Here's how the part is built. I have some questions about the finished solid (model axes, mm). Face numbers are marked on the shaded views. A direction names the side the tool comes from. Give positions to 0.01 mm unless a question says otherwise; leave off trailing zeros. Loops run counter-clockwise (first coordinate to the right, second up) from the corner with the lowest first, then second, coordinate; pieces in that order, holes last. Notation, with made-up numbers: M -25,0 L 24,0 A15 ccw 24,5 Z; hole C -4,76 d8. An arc over 180 degrees is marked long. Answer as CSV lines item,"result". Start each with the question number.
Item 1: For the marked faces 5, 6, 7, 8 and 9, which set-ups out of +Z, -Z, +X, -X, +Y, -Y let a thin tool reach every point of the face, with its end or its side?
Item 2: Will these pins go through, and if not, where does the flat tip stop? P1, Ø2, axis at x = 32, y = 5.5, coming from the -Z side; P2, Ø9, axis at x = -64, y = 13.39, coming from the +Z side; P3, Ø16, axis at x = 16, y = 21.39, coming from the +Z side.
Item 3: I want a section at A-A on x = -16. List the corners of the cut face in (y, z) for me.
Item 4: If I drill on line 1 along X through (y, z) = (39, -4.75); line 2 along Y through (x, z) = (-16, 1.65); line 3 along Y through (x, z) = (64.5, 6.25), over which ranges is the centre line in solid material (lowest first)? Write a range as from..to.
Item 5: I want a section at C-C on x = 26. List the corners of the cut face in (y, z) for me, plus the area to 3 significant figures.
Item 6: If we mould it in two halves opening along X, with no side actions, what happens to the marked faces 1, 2, 3 and 4? For each: released by +X, released by -X, zero draft, split by the parting line, or undercut.
Item 7: I want a section at B-B on z = 5. Give the number of separate pieces and of enclosed holes in the cut face, plus the area to 3 significant figures.
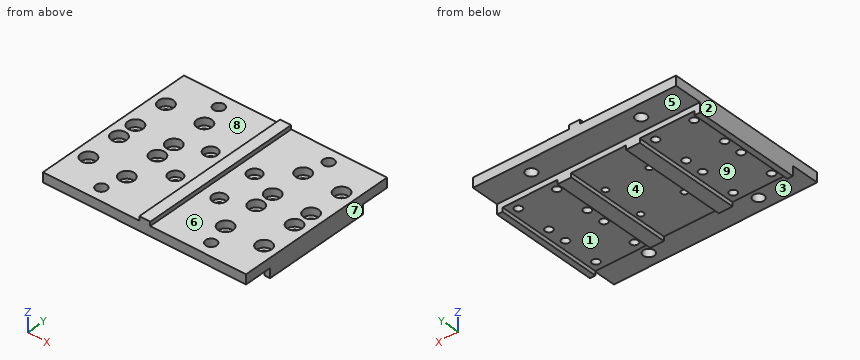
from build123d import *

# Parameters (mm, degrees)
ESQUISSE1_W                                        = 148
ESQUISSE1_H                                        = 120
ESQUISSE1_R                                        = 2.5
ESQUISSE1_R_2                                      = 2
EXTRUSION1_DEPTH                                   = 4
ESQUISSE2_R                                        = 4
ENL_V_MAT_EXTRU_1_DEPTH                            = 100.49847838
ESQUISSE3_W                                        = 148
ESQUISSE3_H                                        = 120
BOSS_EXTRU_1_DEPTH                                 = 3
CHAMBRAGE_POUR_VIS_T_TE_HEXAGONALE_M41_D           = 4.5
CHAMBRAGE_POUR_VIS_T_TE_HEXAGONALE_M41_CBORE_D     = 10
CHAMBRAGE_POUR_VIS_T_TE_HEXAGONALE_M41_CBORE_DEPTH = 4.4
CHAMBRAGE_POUR_VIS_T_TE_HEXAGONALE_M51_D           = 5.5
CHAMBRAGE_POUR_VIS_T_TE_HEXAGONALE_M51_CBORE_D     = 11
CHAMBRAGE_POUR_VIS_T_TE_HEXAGONALE_M51_CBORE_DEPTH = 5.4
ESQUISSE8_R                                        = 4
ENL_V_MAT_EXTRU_2_DEPTH                            = 100.664172098
BOSS_EXTRU_2_START                                 = 4
ESQUISSE9_W                                        = 148
ESQUISSE9_H                                        = 120
ESQUISSE9_R                                        = 2.75
ESQUISSE9_R_2                                      = 2.25
BOSS_EXTRU_2_DEPTH                                 = 4
ESQUISSE11_W                                       = 8
ESQUISSE11_H                                       = 120
BOSS_EXTRU_4_DEPTH                                 = 3
ESQUISSE12_R                                       = 4
ENL_V_MAT_EXTRU_3_DEPTH                            = 100.919703762
ESQUISSE13_R                                       = 2.75
ENL_V_MAT_EXTRU_4_DEPTH                            = 100.919703762
ESQUISSE14_W                                       = 148
ESQUISSE14_H                                       = 20.5
ENL_V_MAT_EXTRU_5_DEPTH                            = 4
ESQUISSE15_W                                       = 4
ESQUISSE15_H                                       = 79
ESQUISSE15_W_2                                     = 10
BOSS_EXTRU_5_DEPTH                                 = 3


with BuildPart() as part:
    # Esquisse1 → Extrusion1 (new body)
    with BuildSketch(Plane.XY):
        with Locations((0, 6.392373056)):
            Rectangle(ESQUISSE1_W, ESQUISSE1_H)
        with Locations((-64, -0.607626944)):
            Circle(ESQUISSE1_R, mode=Mode.SUBTRACT)
        with Locations((-36, 39.392373056)):
            Circle(ESQUISSE1_R, mode=Mode.SUBTRACT)
        with Locations((-64, -26.607626944)):
            Circle(ESQUISSE1_R, mode=Mode.SUBTRACT)
        with Locations((-36, -26.607626944)):
            Circle(ESQUISSE1_R, mode=Mode.SUBTRACT)
        with Locations((36, -0.607626944)):
            Circle(ESQUISSE1_R, mode=Mode.SUBTRACT)
        with Locations((64, -0.607626944)):
            Circle(ESQUISSE1_R, mode=Mode.SUBTRACT)
        with Locations((36, -26.607626944)):
            Circle(ESQUISSE1_R, mode=Mode.SUBTRACT)
        with Locations((64, -26.607626944)):
            Circle(ESQUISSE1_R, mode=Mode.SUBTRACT)
        with Locations((-36, -0.607626944)):
            Circle(ESQUISSE1_R, mode=Mode.SUBTRACT)
        with Locations((-64, 39.392373056)):
            Circle(ESQUISSE1_R, mode=Mode.SUBTRACT)
        with Locations((16, 21.392373056)):
            Circle(ESQUISSE1_R_2, mode=Mode.SUBTRACT)
        with Locations((16, -8.607626944)):
            Circle(ESQUISSE1_R_2, mode=Mode.SUBTRACT)
        with Locations((-16, 21.392373056)):
            Circle(ESQUISSE1_R_2, mode=Mode.SUBTRACT)
        with Locations((-16, -8.607626944)):
            Circle(ESQUISSE1_R_2, mode=Mode.SUBTRACT)
        with Locations((-64, 13.392373056)):
            Circle(ESQUISSE1_R, mode=Mode.SUBTRACT)
        with Locations((-36, 13.392373056)):
            Circle(ESQUISSE1_R, mode=Mode.SUBTRACT)
        with Locations((36, 39.392373056)):
            Circle(ESQUISSE1_R, mode=Mode.SUBTRACT)
        with Locations((36, 13.392373056)):
            Circle(ESQUISSE1_R, mode=Mode.SUBTRACT)
        with Locations((64, 39.392373056)):
            Circle(ESQUISSE1_R, mode=Mode.SUBTRACT)
        with Locations((64, 13.392373056)):
            Circle(ESQUISSE1_R, mode=Mode.SUBTRACT)
    extrude(amount=EXTRUSION1_DEPTH)

    # Esquisse2 → Enlèv. mat.-Extru.1 (cut, through all)
    with BuildSketch(Plane.XY.offset(4)):
        with Locations((-40, 56.392373056)):
            Circle(ESQUISSE2_R)
        with Locations((-40, -43.607626944)):
            Circle(ESQUISSE2_R)
        with Locations((40, 56.392373056)):
            Circle(ESQUISSE2_R)
        with Locations((40, -43.607626944)):
            Circle(ESQUISSE2_R)
    extrude(amount=-ENL_V_MAT_EXTRU_1_DEPTH, mode=Mode.SUBTRACT)

    # Esquisse3 → Boss.-Extru.1 (add)
    with BuildSketch(Plane.XY.offset(4)):
        with Locations((0, 6.392373056)):
            Rectangle(ESQUISSE3_W, ESQUISSE3_H)
    extrude(amount=BOSS_EXTRU_1_DEPTH)

    # Chambrage pour vis à tête hexagonale M41 (through all)
    with Locations(Plane.XY.offset(7)):
        with Locations((-16, 21.392373056), (16, 21.392373056), (16, -8.607626944), (-16, -8.607626944)):
            CounterBoreHole(CHAMBRAGE_POUR_VIS_T_TE_HEXAGONALE_M41_D / 2, CHAMBRAGE_POUR_VIS_T_TE_HEXAGONALE_M41_CBORE_D / 2, CHAMBRAGE_POUR_VIS_T_TE_HEXAGONALE_M41_CBORE_DEPTH)

    # Chambrage pour vis à tête hexagonale M51 (through all)
    with Locations(Plane.XY.offset(7)):
        with Locations((-64, -0.607626944), (-36, -0.607626944), (-36, -26.607626944), (-64, -26.607626944), (36, -0.607626944), (64, -0.607626944), (64, -26.607626944), (36, -26.607626944), (-64, 39.392373056), (-36, 39.392373056), (-64.000489538, 13.39237306), (-36.000489538, 13.39237306), (36, 39.392373056), (64, 39.392373056), (36.038364675, 13.39240136), (64.038364675, 13.392373056)):
            CounterBoreHole(CHAMBRAGE_POUR_VIS_T_TE_HEXAGONALE_M51_D / 2, CHAMBRAGE_POUR_VIS_T_TE_HEXAGONALE_M51_CBORE_D / 2, CHAMBRAGE_POUR_VIS_T_TE_HEXAGONALE_M51_CBORE_DEPTH)

    # Esquisse8 → Enlèv. mat.-Extru.2 (cut, through all)
    with BuildSketch(Plane(origin=(0, 0, 0), x_dir=(-1, 0, 0), z_dir=(0, 0, -1))):
        with Locations(Location((40, -43.607626944, 0), (0, 0, 180))):
            Circle(ESQUISSE8_R)
        with Locations(Location((40, 56.392373056, 0), (0, 0, 180))):
            Circle(ESQUISSE8_R)
        with Locations(Location((-40, 56.392373056, 0), (0, 0, 180))):
            Circle(ESQUISSE8_R)
        with Locations(Location((-40, -43.607626944, 0), (0, 0, 180))):
            Circle(ESQUISSE8_R)
    extrude(amount=-ENL_V_MAT_EXTRU_2_DEPTH, mode=Mode.SUBTRACT)

    # Esquisse9 → Boss.-Extru.2 (add)
    with BuildSketch(Plane(origin=(0, 0, 0), x_dir=(-1, 0, 0), z_dir=(0, 0, -1)).offset(BOSS_EXTRU_2_START)):
        with Locations((0, 6.392373056)):
            Rectangle(ESQUISSE9_W, ESQUISSE9_H)
        with Locations(Location((-64, -0.607626944, 0), (0, 0, 180))):
            Circle(ESQUISSE9_R, mode=Mode.SUBTRACT)
        with Locations(Location((-64, -26.607626944, 0), (0, 0, 180))):
            Circle(ESQUISSE9_R, mode=Mode.SUBTRACT)
        with Locations(Location((-36, -0.607626944, 0), (0, 0, 180))):
            Circle(ESQUISSE9_R, mode=Mode.SUBTRACT)
        with Locations(Location((-36, -26.607626944, 0), (0, 0, 180))):
            Circle(ESQUISSE9_R, mode=Mode.SUBTRACT)
        with Locations(Location((-16, 21.392373056, 0), (0, 0, 180))):
            Circle(ESQUISSE9_R_2, mode=Mode.SUBTRACT)
        with Locations(Location((16, 21.392373056, 0), (0, 0, 180))):
            Circle(ESQUISSE9_R_2, mode=Mode.SUBTRACT)
        with Locations(Location((-16, -8.607626944, 0), (0, 0, 180))):
            Circle(ESQUISSE9_R_2, mode=Mode.SUBTRACT)
        with Locations(Location((16, -8.607626944, 0), (0, 0, 180))):
            Circle(ESQUISSE9_R_2, mode=Mode.SUBTRACT)
        with Locations(Location((36, -0.607626944, 0), (0, 0, 180))):
            Circle(ESQUISSE9_R, mode=Mode.SUBTRACT)
        with Locations(Location((64, -0.607626944, 0), (0, 0, 180))):
            Circle(ESQUISSE9_R, mode=Mode.SUBTRACT)
        with Locations(Location((36, -26.607626944, 0), (0, 0, 180))):
            Circle(ESQUISSE9_R, mode=Mode.SUBTRACT)
        with Locations(Location((64, -26.607626944, 0), (0, 0, 180))):
            Circle(ESQUISSE9_R, mode=Mode.SUBTRACT)
    extrude(amount=-BOSS_EXTRU_2_DEPTH)

    # Esquisse11 → Boss.-Extru.4 (add)
    with BuildSketch(Plane.XY.offset(7)):
        with Locations((0.163625215, 6.392373056)):
            Rectangle(ESQUISSE11_W, ESQUISSE11_H)
    extrude(amount=BOSS_EXTRU_4_DEPTH)

    # Esquisse12 → Enlèv. mat.-Extru.3 (cut, through all)
    with BuildSketch(Plane.XY):
        with Locations((-40, 56.392373056)):
            Circle(ESQUISSE12_R)
        with Locations((40, 56.392373056)):
            Circle(ESQUISSE12_R)
        with Locations((40, -43.607626944)):
            Circle(ESQUISSE12_R)
        with Locations((-40, -43.607626944)):
            Circle(ESQUISSE12_R)
    extrude(amount=-ENL_V_MAT_EXTRU_3_DEPTH, mode=Mode.SUBTRACT)

    # Esquisse13 → Enlèv. mat.-Extru.4 (cut, through all)
    with BuildSketch(Plane.XY):
        with Locations((-64, 39.392373056)):
            Circle(ESQUISSE13_R)
        with Locations((-36, 39.392373056)):
            Circle(ESQUISSE13_R)
        with Locations((-36.000489538, 13.39237306)):
            Circle(ESQUISSE13_R)
        with Locations((-64.000489538, 13.39237306)):
            Circle(ESQUISSE13_R)
        with Locations((36, 39.392373056)):
            Circle(ESQUISSE13_R)
        with Locations((64, 39.392373056)):
            Circle(ESQUISSE13_R)
        with Locations((36.038364675, 13.39240136)):
            Circle(ESQUISSE13_R)
        with Locations((64.038364675, 13.392373056)):
            Circle(ESQUISSE13_R)
    extrude(amount=-ENL_V_MAT_EXTRU_4_DEPTH, mode=Mode.SUBTRACT)

    # Esquisse14 → Enlèv. mat.-Extru.5 (cut)
    with BuildSketch(Plane(origin=(0, 0, -4), x_dir=(-1, 0, 0), z_dir=(0, 0, -1))):
        with Locations((0, -43.357626944)):
            Rectangle(ESQUISSE14_W, ESQUISSE14_H)
        with Locations((0, 56.142373056)):
            Rectangle(ESQUISSE14_W, ESQUISSE14_H)
    extrude(amount=-ENL_V_MAT_EXTRU_5_DEPTH, mode=Mode.SUBTRACT)

    # Esquisse15 → Boss.-Extru.5 (add)
    with BuildSketch(Plane(origin=(0, 0, -4), x_dir=(-1, 0, 0), z_dir=(0, 0, -1))):
        with Locations((-72, 6.392373056)):
            Rectangle(ESQUISSE15_W, ESQUISSE15_H)
        with Locations((-25, 6.392373056)):
            Rectangle(ESQUISSE15_W_2, ESQUISSE15_H)
        with Locations((25, 6.392373056)):
            Rectangle(ESQUISSE15_W_2, ESQUISSE15_H)
        with Locations((72, 6.392373056)):
            Rectangle(ESQUISSE15_W, ESQUISSE15_H)
    extrude(amount=BOSS_EXTRU_5_DEPTH)


solid = part.part
Result:
1,face 5,"-Z, +X, -X, +Y"
1,face 6,"+Z, +X, +Y, -Y"
1,face 7,"+Z, -Z, +X, +Y, -Y"
1,face 8,"+Z, -X, +Y, -Y"
1,face 9,"-Z, +Y, -Y"
2,P1,"z = -4"
2,P2,"z = 1.6"
2,P3,"z = 7"
3,outline,"M -53.61,0 L -33.11,0 L -33.11,-4 L -10.86,-4 L -10.86,2.6 L -13.61,2.6 L -13.61,7 L -53.61,7 Z; M -6.36,-4 L 19.14,-4 L 19.14,2.6 L 16.39,2.6 L 16.39,7 L -3.61,7 L -3.61,2.6 L -6.36,2.6 Z; M 23.64,-4 L 45.89,-4 L 45.89,0 L 66.39,0 L 66.39,7 L 26.39,7 L 26.39,2.6 L 23.64,2.6 Z"
4,line 1,"-74..-70, -30..-20, 20..30, 70..74"
4,line 2,"-53.61..-10.86, -6.36..19.14, 23.64..66.39"
4,line 3,"-53.61..-32.08, -21.13..-6.08, 4.87..7.91, 18.87..33.92, 44.87..66.39"
5,outline,"M -53.61,0 L -33.11,0 L -33.11,-7 L 45.89,-7 L 45.89,0 L 66.39,0 L 66.39,7 L -53.61,7 Z"
5,area,"1,390 mm^2"
6,face 1,"undercut"
6,face 2,"released by -X"
6,face 3,"zero draft"
6,face 4,"undercut"
7,separate pieces,"1"
7,enclosed holes,"24"
7,area,"15,700 mm^2"
